Source: CAD feature listing. Evaluate the final solid. Frame: model axes, mm. A direction names the side the tool comes from. Round coordinates to 2 decimals unless told otherwise and drop trailing zeros. Loops run counter-clockwise (first coordinate to the right, second up) from the corner with the lowest first, then second, coordinate; pieces in that order, holes last. Notation, with made-up numbers: (66, 73.25) -> (114, 73.25) arc R19 cw to (114, 83.25) -> close; hole circle Ø4 at (-19.75, 6). An arc over 180 degrees is marked (long way). Put each result on its own line as item: value. Start each with the question number.
1. Material intervals for L1, parallel to Z at x = 64.5, y = -12; L2, parallel to Y at x = 17, z = -43; L3, parallel to X at y = 11, z = -21, sorted ascending.
2. Cut plane B-B (y = -23). Return the cut outline in (x, z).
3. Draft query along X for faces 1 (the flat face through (12, -4.751, -25)), 2 (the flat face through (13, -29.751, -25)), 3 (the flat face through (75.849, -7, -45)), 4 (the flat face through (-8.151, 5, -25)). Return one class per face: pulls with the +X half, pulls with the -X half, needs draft (parallel to the pull), parting line crosses it, or undercut.
4. Cut plane C-C (z = -27.5). Return the cut outline in (x, y).
5. Cut plane A-A (y = 2). Return the cut outline in (x, z), then the cut area to 3 significant figures.
6. Set-up query: faces 5 (the flat face through (-46, -7, -10)), 6 (the flat face through (70, -7, -10)), 7 (the flat face through (31.849, 5, -25)). Return all of +Z, -Z, +X, -X, +Y, -Y with unobstructed straight access to the full face (end or side cutting, diameter ignored); none if empty.
7. Contact query for flat-ended pins moving along their axis: pin 1 (3 mm diameter, centred on y = 3, z = -35.5, fed in from +X); pin 2 (10 mm diameter, centred on x = -7, z = -44, fed in from +Y); pin 3 (2 mm diameter, centred on y = -7, z = -27.5, fed in from +X); pin 4 (16 mm diameter, centred on y = 6, z = -19, fed in from -X). Output: stop coordinate, or through.
8. Cut plane D-D (x = 25.5). Return the cut outline in (y, z).
Autodesk Inventor part; units mm, degrees
ref_plane "YZ Plane" through (0, 0, 0) normal (1, 0, 0) x (0, 1, 0)
ref_plane "XZ Plane" through (0, 0, 0) normal (0, 1, 0) x (-1, 0, 0)
ref_plane "XY Plane" through (0, 0, 0) normal (0, 0, 1) x (1, 0, 0)
sketch "Sketch1" plane through (0, 0, 0) normal (0, 0, 1) x (1, 0, 0)
  line L0 (-52.1514, 15.2486) -> (75.8486, 15.2486)
  line L1 (75.8486, 15.2486) -> (75.8486, -29.7514)
  line L2 (75.8486, -29.7514) -> (-52.1514, -29.7514)
  line L3 (-52.1514, -29.7514) -> (-52.1514, 15.2486)
  point P0 (0, 0)
  dimension "d0" = 128
  dimension "d1" = 128
  dimension "d2" = 45
extrude "Extrusion1" add sketch "Sketch1" against normal blind 50
ref_plane "Work Plane1" through (0, 0, -50) normal (0, 0, -1) x (-1, 0, 0)
sketch "Sketch2" plane through (0, 0, -50) normal (0, 0, -1) x (-1, 0, 0)
  line L0 (52.1514, 15.2486) -> (-75.8486, 15.2486)
  line L1 (-31.8486, 15.2486) -> (-31.8486, -4.7514)
  line L2 (-31.8486, -4.7514) -> (8.1514, -4.7514)
  line L3 (8.1514, -4.7514) -> (8.1514, 15.2486)
  point P0 (0, 0)
  dimension "d6" = 44
  dimension "d7" = 44
  dimension "d8" = 20
extrude "Extrusion2" cut sketch "Sketch2" against normal blind 50
sketch "Sketch3" plane through (75.8486, -29.7514, 0) normal (1, 0, 0) x (0, 0, -1)
  line L0 (0, 45) -> (50, 45)
  line L1 (10, 45) -> (10, 29.7514)
  point P0 (0, 29.7514)
  point P1 (40, 45)
  dimension "d11" = 10
  dimension "d12" = 10
sketch "Sketch4" plane through (75.8486, 15.2486, 0) normal (0, 1, 0) x (1, 0, 0)
  line L0 (0, 0) -> (0, 50)
  line L1 (0, 50) -> (-128, 50)
  line L2 (0, 10) -> (-12, 10)
  line L3 (-12, 10) -> (-11.4432, 40.2365)
  line L4 (-11.4432, 40.2365) -> (0.5568, 40.0155)
  point P0 (-75.8486, 0)
  point P1 (0, 40.0258)
  dimension "d13" = 10
  dimension "d14" = 10
  dimension "d15" = 12
  dimension "d16" = 12
extrude "Extrusion3" cut sketch "Sketch4" against normal blind 50
sketch "Sketch5" plane through (31.8486, 15.2486, 0) normal (0, 1, 0) x (1, 0, 0)
  line L0 (-84, 0) -> (-84, 50)
  line L1 (44, 50) -> (-84, 50)
  line L2 (-84, 10) -> (-72, 10)
  line L3 (-72, 10) -> (-72, 40)
  line L4 (-72, 40) -> (-84, 40)
  point P0 (-31.8486, 0)
  dimension "d19" = 10
  dimension "d20" = 10
  dimension "d21" = 12
  dimension "d22" = 12
extrude "Extrusion4" cut sketch "Sketch5" against normal blind 50
Solution:
1. L1: z = -50 to -40.23, -10 to 0
1. L2: y = -29.75 to -4.75
1. L3: x = -40.15 to -8.15, 31.85 to 64.05
2. outline: (-52.15, -50) -> (75.85, -50) -> (75.85, -40.03) -> (64.41, -40.24) -> (63.85, -10) -> (75.85, -10) -> (75.85, 0) -> (-52.15, 0) -> (-52.15, -10) -> (-40.15, -10) -> (-40.15, -40) -> (-52.15, -40) -> close
3. face 1: undercut
3. face 2: needs draft
3. face 3: pulls with the +X half
3. face 4: undercut
4. outline: (-40.15, -29.75) -> (64.17, -29.75) -> (64.17, 15.25) -> (31.85, 15.25) -> (31.85, -4.75) -> (-8.15, -4.75) -> (-8.15, 15.25) -> (-40.15, 15.25) -> close
5. outline: (-52.15, -50) -> (-8.15, -50) -> (-8.15, 0) -> (-52.15, 0) -> (-52.15, -10) -> (-40.15, -10) -> (-40.15, -40) -> (-52.15, -40) -> close; (31.85, -50) -> (75.85, -50) -> (75.85, -40.03) -> (64.41, -40.24) -> (63.85, -10) -> (75.85, -10) -> (75.85, 0) -> (31.85, 0) -> close
5. area: 3,690 mm^2
6. face 5: -X, +Y, -Y
6. face 6: +X, +Y, -Y
6. face 7: +Z, -Z, +Y
7. pin 1: stops at x = 64.35
7. pin 2: stops at y = 15.25
7. pin 3: stops at x = 64.19
7. pin 4: stops at x = -40.15
8. outline: (-29.75, -50) -> (-4.75, -50) -> (-4.75, 0) -> (-29.75, 0) -> close
